Input: dimensioned drawing with shaded views. Units: mm. Origin: part minimum x, y, z. A direction names the side the tool comes from. Round coordinates to 2 decimals unless told otherwise and drop trailing zeros. Loops run counter-clockwise (first coordinate to the right, second up) from the corner with the lowest first, then second, coordinate; pieces in that order, holes last.
Item 1: Section query B-B on y = 15. Return loops of the section in (x, z), then the cut area to 4 significant figures.
Item 2: Pull-direction query (Y, two-part tool) for the marked faces 3 and 4; classes: released by +Y, released by -Y, zero draft, split by the parting line, or undercut.
Item 3: Ray query, L1, parallel to Y at x = 15, z = 3; L2, parallel to Z at x = 22.5, y = 19.25. Return the intervals inside material, ascending.
Item 4: Section query A-A on x = 18. Return loops of the section in (y, z), then the cut area to 3 significant figures.
Item 5: Section query D-D on x = 25. Return loops of the section in (y, z).
Item 6: Section query C-C on z = 2.5. Return loops of the section in (x, y).
Item 7: First-contact query: P1, Ø1.6, axis at x = 41, z = 1, coming from the -Y side; P2, Ø0.6, axis at x = 11.5, z = 2.5, coming from the -Y side; P3, Ø1, axis at y = 5.5, z = 1, coming from the +X side. Flat tips, straight axial feed; report the tip coordinate or a pass-through.
Item 8: Access query for the marked faces 1 and 2. Directions: +Z, -Z, +X, -X, +Y, -Y. A direction counts if a zero-diameter tool reaches every point of the face in a straight line with its end or side. Return the directions, or none.
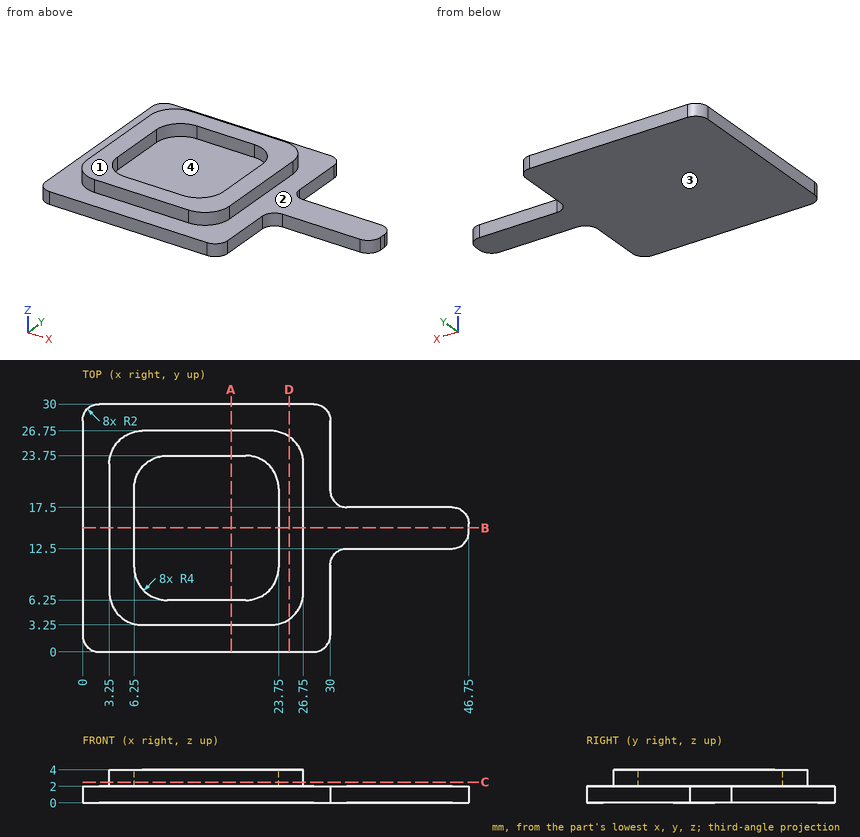
Data:
1. outline: (0, 0) - (46.75, 0) - (46.75, 2) - (26.75, 2) - (26.75, 4) - (23.75, 4) - (23.75, 2) - (6.25, 2) - (6.25, 4) - (3.25, 4) - (3.25, 2) - (0, 2) - close
1. area: 105.5 mm2
2. face 3: zero draft
2. face 4: undercut
3. L1: y = 3.25 to 6.25, 23.75 to 26.75
3. L2: z = 0 to 2
4. outline: (0, 0) - (30, 0) - (30, 2) - (26.75, 2) - (26.75, 4) - (23.75, 4) - (23.75, 2) - (6.25, 2) - (6.25, 4) - (3.25, 4) - (3.25, 2) - (0, 2) - close
4. area: 72.0 mm2
5. outline: (0, 0) - (30, 0) - (30, 2) - (26.06, 2) - (26.06, 4) - (3.94, 4) - (3.94, 2) - (0, 2) - close
6. outline: (3.25, 7.25) arc R4 ccw to (7.25, 3.25) - (22.75, 3.25) arc R4 ccw to (26.75, 7.25) - (26.75, 22.75) arc R4 ccw to (22.75, 26.75) - (7.25, 26.75) arc R4 ccw to (3.25, 22.75) - close; hole (6.25, 10.25) arc R4 ccw to (10.25, 6.25) - (19.75, 6.25) arc R4 ccw to (23.75, 10.25) - (23.75, 19.75) arc R4 ccw to (19.75, 23.75) - (10.25, 23.75) arc R4 ccw to (6.25, 19.75) - close
7. P1: stops at y = 12.5
7. P2: stops at y = 3.25
7. P3: stops at x = 30
8. face 1: +Z, +X, -X, +Y, -Y
8. face 2: +Z
